from build123d import *

# Parameters (mm, degrees)
CROQUIS1_R              = 2
SALIENTE_EXTRUIR1_DEPTH = 10
CROQUIS3_R              = 2
CORTAR_EXTRUIR1_DEPTH   = 5


with BuildPart() as part:
    # Croquis1 → Saliente-Extruir1 (new body)
    with BuildSketch(Plane(origin=(0, 0, 0), x_dir=(1, 0, 0), z_dir=(0, 1, 0))):
        with BuildLine():
            Line((0.204691251, -6.496776238), (-39.795308749, -6.496776238))
            Line((-39.795308749, -6.496776238), (-47.602797524, -13.442682877))
            Line((-47.602797524, -13.442682877), (-47.602797524, -22.442682877))
            ThreePointArc((-47.602797524, -22.442682877), (-52.352797524, -27.192682877), (-57.102797524, -22.442682877))
            Line((-57.102797524, -22.442682877), (-57.102797524, -6.542682877))
            Line((-57.102797524, -6.542682877), (-40.113440642, 5.800807421))
            Line((-40.113440642, 5.800807421), (-0.113440642, 6.499010019))
            ThreePointArc((-0.113440642, 6.499010019), (6.498053307, 0.159069868), (0.204691251, -6.496776238))
        make_face()
        with Locations(Location((0, 0, 0), (0, 0, 270))):
            Circle(CROQUIS1_R, mode=Mode.SUBTRACT)
    extrude(amount=SALIENTE_EXTRUIR1_DEPTH)

    # Croquis3 → Cortar-Extruir1 (cut)
    with BuildSketch(Plane.XZ):
        with BuildLine():
            Line((0.204691251, 6.496776238), (-6.795308749, 6.496776238))
            Line((-6.795308749, 6.496776238), (-6.795308749, -6.382377577))
            Line((-6.795308749, -6.382377577), (-0.113440642, -6.499010019))
            ThreePointArc((-0.113440642, -6.499010019), (6.498053307, -0.159069868), (0.204691251, 6.496776238))
        make_face()
        with Locations(Location((0, 0, 0), (0, 0, 270))):
            Circle(CROQUIS3_R, mode=Mode.SUBTRACT)
    extrude(amount=-CORTAR_EXTRUIR1_DEPTH, mode=Mode.SUBTRACT)


solid = part.part
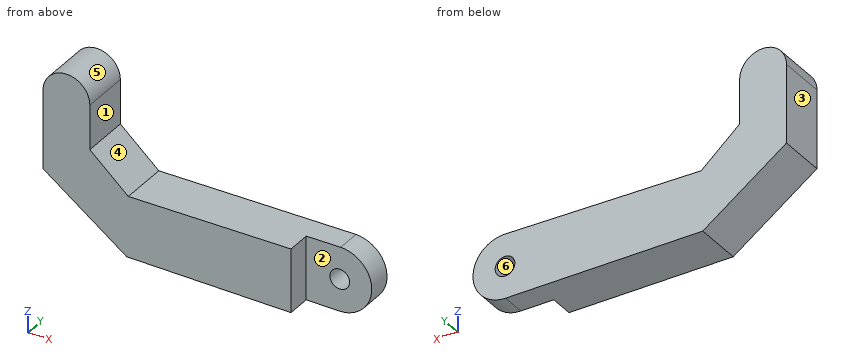
For this review, take the finished solid that the model builds, in its own axes (mm). Face numbers are marked on the shaded views. A direction names the side the tool comes from. Give positions to 0.01 mm unless a question says otherwise; leave off trailing zeros. Order: outer loops, then holes, each group sorted by start corner. A loop starts at its lowest first (then second) coordinate and runs counter-clockwise, first axis right, second up. Notation, with made-up numbers: M 30.5,21.25 L 37.5,21.25 A28 cw 37.5,55.25 Z; hole C -32,34 d4. An arc over 180 degrees is marked long. Answer in a Markdown table with one row per item. Add a question column.
(1) Consider section C-C on x = -49.5. State the section outline as (y, z) points.
(2) Wall thickness on probe 1 along X at (y, z) = (6.15, 0); probe 2 along X at (y, z) = (9, 19); probe 3 along X at (y, z) = (8.5, -1): over which ranges is each line inside the solid? List them lowest first. Write a range as [from, to].
(3) Consider section A-A on y = 2.25. State the section outline as (x, z) points, and give its area (3 significant figures).
(4) For pin 1 (4 mm diameter, centred on x = 0.5, z = -2.5, fed in from -Y); pin 2 (5 mm diameter, centred on x = -19.5, y = 6.5, fed in from +Z); pin 3 (2 mm diameter, centred on y = 3.5, z = -1, fed in from -X), all flat-tipped, find the tip position at first contact; note any pin that passes through.
(5) Consider section B-B on z = 0. State the section outline as (x, y) points.
(6) Mouldability with a two-part tool opening along X and no side actions: class the marked faces 4, 5 and 6 as +X half, -X half, draft (parallel to the pull), parting line (faces both ways), or undercut.
(7) Consider section D-D on z = 9. State the section outline as (x, y) points.
(8) For the marked faces 1, 2 and 3, list the 3-axis set-ups (+Z, -Z, +X, -X, +Y, -Y) from which the entire face can be reached by the end or side of a thin tool; tool diameter is ignored.
Evaluation:
| question | item | result |
|---|---|---|
| 1 | outline | M 0,1.02 L 10,1.02 L 10,26.24 L 0,26.24 Z |
| 2 | probe 1 | x = [-48.1, -2], [2, 6.5] |
| 2 | probe 2 | x = [-57.1, -47.6] |
| 2 | probe 3 | x = [-46.72, -1.73], [1.73, 6.42] |
| 3 | outline | M -57.1,6.54 L -40.11,-5.8 L -6.8,-6.38 L -6.8,6.5 L -39.8,6.5 L -47.6,13.44 L -47.6,22.44 A4.75 ccw -57.1,22.44 Z |
| 3 | area | 738 mm^2 |
| 4 | pin 1 | stops at y = 5 |
| 4 | pin 2 | stops at z = 6.5 |
| 4 | pin 3 | stops at x = -48.1 |
| 5 | outline | M -48.1,0 L -6.8,0 L -6.8,5 L -2,5 L -2,10 L -48.1,10 Z; M 2,5 L 6.5,5 L 6.5,10 L 2,10 Z |
| 6 | face 4 | +X half |
| 6 | face 5 | parting line |
| 6 | face 6 | undercut |
| 7 | outline | M -57.1,0 L -42.61,0 L -42.61,10 L -57.1,10 Z |
| 8 | face 1 | +Z, +X, +Y, -Y |
| 8 | face 2 | +Z, -Z, +X, -Y |
| 8 | face 3 | +Z, -Z, -X, +Y, -Y |
